Geometry: final body of the model. Coordinates: model frame, mm. A direction names the side the tool comes from. Give positions to 0.01 mm unless a question says otherwise; leave off trailing zeros. Write each loop counter-clockwise with the first axis right and the second up, starting at its lowest first coordinate (ties: lowest second). Pieces come first, ordered by that corner, then holes.
Q1. Pin query (flat end, axial travel): pin 1 Ø2 at (x, z) = (20.5, 7) entering from +Y; pin 2 Ø1.3 at (x, z) = (21, 7) entering from -Y; pin 3 Ø3 at (x, y) = (23.5, 14) entering from +Z; pin 4 Ø1 at (y, z) = (29.5, 7) entering from +X. Return the tip coordinate at first contact, or that it passes through.
Q2. Section A-A (z = 6.75). Return the cut outline in (x, y) (3 decimals).
Q3. Mould query, pull axis Y, two halves, no side actions, for faces 1 (the cylindrical face through (9.61, 3.81, 2.58)), 2 (the flat face through (22.86, 11, 9)), 3 (the flat face through (19, 16.932, 6)), 4 (the flat face through (17.44, 40.78, 6.33)). Classes: +Y half, -Y half, draft (parallel to the pull), parting line (faces both ways), or undercut.
Q4. Reachability of faces 5 (the flat face through (19, 6.35, 6)), 6 (the flat face through (19, 12.446, 9)), 7 (the flat face through (35, 0, 3)) from +Z, -Z, +X, -X, +Y, -Y: full face, straight path, thin tool, end or side. Return the list, or none.
Q5. Line query: line 1 (X direction, y = 3.5, z = 5); line 2 (Z direction, x = 25.5, y = 10); line 3 (Z direction, x = 14.5, y = 42.5). Output: solid intervals per line, ascending.
Q6. Section C-C (y = 48). Return the cut outline in (x, z), plus the area to 3 significant figures.
Q7. Section D-D (x = 11). Return the cut outline in (y, z).
Q8. Section B-B (z = 3). Return the cut outline in (x, y) (3 decimals), plus the area to 3 significant figures.
from build123d import *

# Parameters (mm, degrees)
F1_DEPTH = 5.08
F2_DEPTH = 7.62
F0_W     = 3.81
F0_H     = 3.81
F3_DEPTH = 10.16
F4_DEPTH = 7.62
F5_D     = 7.62
F6_D     = 7.62


with BuildPart() as f1:
    # F0 (on Top) → F1 (new body)
    with BuildSketch(Plane.XY):
        Polygon((9.825618, 16.93164), (0, 0), (19.05, 0), (19.05, 6.35), (10.16, 6.35), (16.300643, 16.93164), align=None)
        Polygon((19.05, 6.35), (19.05, 0), (38.1, 0), (28.274382, 16.93164), (21.799357, 16.93164), (27.94, 6.35), align=None)
        Polygon((21.799357, 16.93164), (28.274382, 16.93164), (22.225, 50.8), (19.05, 30.48), (19.05, 16.93164), align=None)
        Polygon((15.875, 50.8), (9.825618, 16.93164), (16.300643, 16.93164), (19.05, 16.93164), (19.05, 30.48), align=None)
        Polygon((19.05, 68.575706), (15.875, 50.8), (19.05, 50.8), (22.225, 50.8), align=None)
        Polygon((22.225, 50.8), (19.05, 50.8), (19.05, 30.48), align=None)
        Polygon((19.05, 50.8), (15.875, 50.8), (19.05, 30.48), align=None)
    extrude(amount=F1_DEPTH)

    # F0 (on Top) → F2 (join)
    with BuildSketch(Plane.XY):
        Polygon((10.16, 6.35), (19.05, 6.35), (19.05, 8.636), (15.24, 8.636), (15.24, 12.446), (19.05, 12.446), (19.05, 16.93164), (16.300643, 16.93164), align=None)
        Polygon((19.05, 8.636), (19.05, 6.35), (27.94, 6.35), (21.799357, 16.93164), (19.05, 16.93164), (19.05, 12.446), (22.86, 12.446), (22.86, 8.636), align=None)
    extrude(amount=F2_DEPTH)

    # F0 (on Top) → F3 (join)
    with BuildSketch(Plane.XY):
        with Locations((17.145, 10.541)):
            Rectangle(F0_W, F0_H)
        with Locations((20.955, 10.541)):
            Rectangle(F0_W, F0_H)
    extrude(amount=F3_DEPTH)

    # F0 (on Top) → F4 (join)
    with BuildSketch(Plane.XY):
        Polygon((19.05, 50.8), (15.875, 50.8), (19.05, 30.48), align=None)
        Polygon((22.225, 50.8), (19.05, 50.8), (19.05, 30.48), align=None)
    extrude(amount=F4_DEPTH)

    # F5 (through all)
    with Locations(Plane(origin=(0, 0, 0), x_dir=(1, 0, 0), z_dir=(0, 0, -1))):
        with Locations((19.05, 0)):
            Hole(F5_D / 2)

    # F6 (through all)
    with Locations(Plane(origin=(0, 0, 0), x_dir=(1, 0, 0), z_dir=(0, 0, -1))):
        with Locations((9.525, 0), (28.575, 0)):
            Hole(F6_D / 2)


solid = f1.part
Computed:
1. pin 1: stops at y = 50.8
1. pin 2: stops at y = 6.35
1. pin 3: stops at z = 7.62
1. pin 4: passes through
2. outline: (10.16, 6.35) - (27.94, 6.35) - (21.799, 16.932) - (16.301, 16.932) - close; (15.875, 50.8) - (19.05, 30.48) - (22.225, 50.8) - close
3. face 1: -Y half
3. face 2: draft
3. face 3: undercut
3. face 4: undercut
4. face 5: +Z, +X, -X, -Y
4. face 6: +Z, +X, -X, +Y
4. face 7: +Z, -Z, +X, -X, -Y
5. line 1: x = 2.03 to 8.02, 11.03 to 17.54, 20.56 to 27.07, 30.08 to 36.07
5. line 2: z = 0 to 7.62
5. line 3: z = 0 to 5.08
6. outline: (15.37, 0) - (22.73, 0) - (22.73, 5.08) - (21.79, 5.08) - (21.79, 7.62) - (16.31, 7.62) - (16.31, 5.08) - (15.37, 5.08) - close
6. area: 51.2 mm2
7. outline: (3.51, 0) - (23.51, 0) - (23.51, 5.08) - (7.8, 5.08) - (7.8, 7.62) - (6.35, 7.62) - (6.35, 5.08) - (3.51, 5.08) - close
8. outline: (0, 0) - (5.715, 0) arc R3.81 cw to (13.335, 0) - (15.24, 0) arc R3.81 cw to (22.86, 0) - (24.765, 0) arc R3.81 cw to (32.385, 0) - (38.1, 0) - (28.274, 16.932) - (19.05, 68.576) - (9.826, 16.932) - close
8. area: 887 mm2
